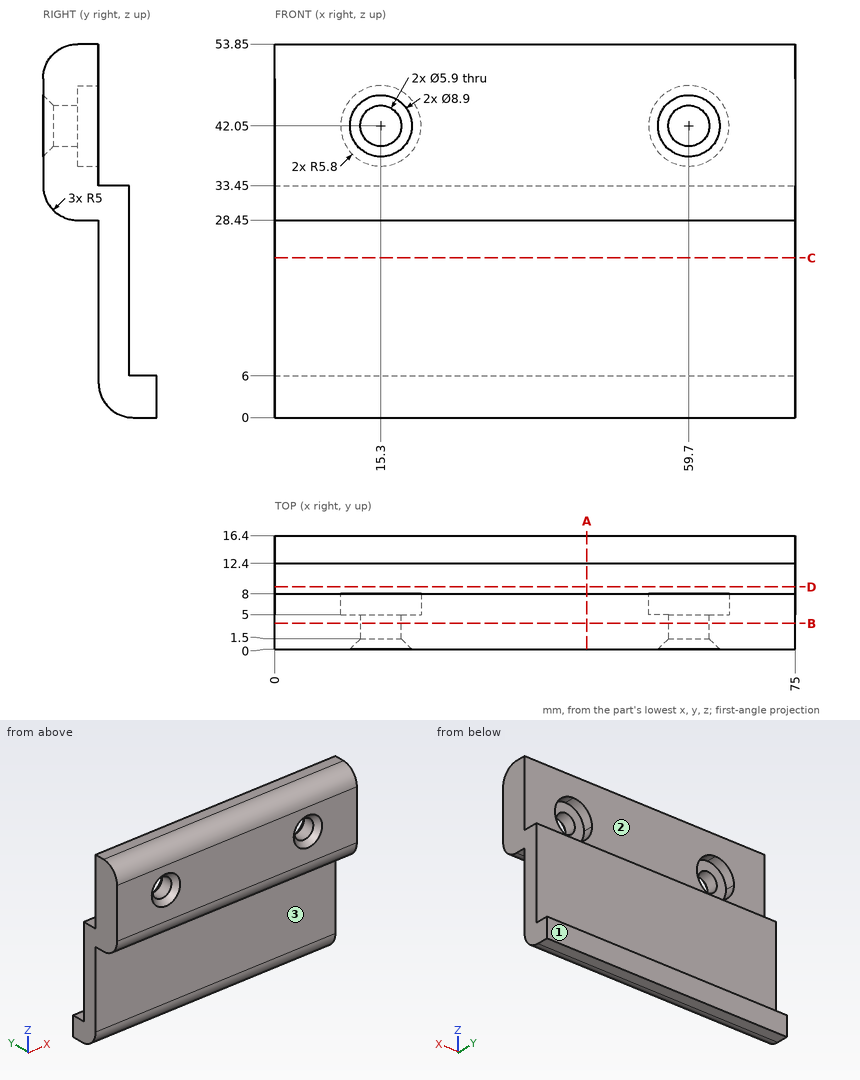
Geometry: see drawing. Coordinates: mm, zero at the bounding-box minimum. A direction names the side the tool comes from. Round coordinates to 2 decimals unless told otherwise and drop trailing zeros. Loops run counter-clockwise (first coordinate to the right, second up) from the corner with the lowest first, then second, coordinate; pieces in that order, holes last. Notation, with made-up numbers: (78, 66.25) -> (82, 66.25) arc R29 ccw to (82, 87.25) -> close; hole circle Ø10 at (38, 9). An arc over 180 degrees is marked (long way). One line per question, with ' | ' between items. Start each with the question number.
1. Section D-D on y = 9. Output: boundary loops of the cut face in (x, z), and give its area (3 significant figures).
2. Section A-A on x = 45. Output: boundary loops of the cut face in (y, z).
3. Contact query for flat-ended pins moving along their axis: pin 1 (1.5 mm diameter, centred on x = 27, y = 9.5, fed in from -Z); pin 2 (8 mm diameter, centred on x = 50.5, z = 14, fed in from +Y); pin 3 (0.9 mm diameter, centred on x = 46.5, y = 7, fed in from -Z). Output: stop coordinate, or through.
4. Set-up query: the marked faces 1, 2 and 3. Return all of +Z, -Z, +X, -X, +Y, -Y with unobstructed straight access to the full face (end or side cutting, diameter ignored); none if empty.
5. Section B-B on y = 3.75. Output: boundary loops of the cut face in (x, z).
6. Section C-C on z = 23. Output: boundary loops of the cut face in (x, y), and give its area (3 significant figures).
7. Line query: line 1 along X through (y, z) = (6.75, 37.5); line 2 along Y through (x, z) = (30, 49); line 3 along Z through (x, y) = (14, 13.5). Output: solid intervals per line, ascending. Write a range as [from, to].
Returned:
1) outline: (0, 2) -> (75, 2) -> (75, 33.45) -> (0, 33.45) -> close | area: 2,360 mm2
2) outline: (0, 33.45) arc R5 ccw to (5, 28.45) -> (8, 28.45) -> (8, 5) arc R5 ccw to (13, 0) -> (16.4, 0) -> (16.4, 6) -> (12.4, 6) -> (12.4, 33.45) -> (8, 33.45) -> (8, 53.85) -> (5, 53.85) arc R5 ccw to (0, 48.85) -> close
3) pin 1: stops at z = 0.82 | pin 2: stops at y = 12.4 | pin 3: stops at z = 28.45
4) face 1: +Z, -Z, +X, -X, +Y | face 2: +Z, +X, -X, +Y | face 3: -Z, +X, -X, -Y
5) outline: (0, 28.61) -> (75, 28.61) -> (75, 53.69) -> (0, 53.69) -> close; hole circle Ø5.9 at (15.3, 42.05); hole circle Ø5.9 at (59.7, 42.05)
6) outline: (0, 8) -> (75, 8) -> (75, 12.4) -> (0, 12.4) -> close | area: 330 mm2
7) line 1: x = [0, 11.7], [18.9, 56.1], [63.3, 75] | line 2: y = [0, 8] | line 3: z = [0, 6]
